Could you check a few things on this model? Use its own coordinates, in mm. A direction names the side the tool comes from. Coordinates: 2 decimals unless noted, no trailing zeros. Order: outer loops, then holes, each group sorted by start corner. A loop starts at its lowest first (then second) coordinate and runs counter-clockwise, first axis right, second up. Notation, with made-up numbers: (-2.75, -17) - (35.25, -17) arc R18 cw to (35.25, 17) - close; hole circle Ø7 at (3, -30.5). An arc over 180 degrees is marked (long way). One line per item, written item: value.
from build123d import *

# Parameters (mm, degrees)
SKETCH1_R           = 5.1435
BOSS_EXTRUDE1_DEPTH = 10.3
BOSS_EXTRUDE2_DEPTH = 7.5
SKETCH3_R           = 10.75
BOSS_EXTRUDE3_DEPTH = 10.3
SKETCH4_R           = 9.525
BOSS_EXTRUDE4_DEPTH = 1.5
SKETCH5_R           = 8.255
BOSS_EXTRUDE5_DEPTH = 12
SKETCH6_R           = 10
BOSS_EXTRUDE6_DEPTH = 11.4
SKETCH7_R           = 4.3053
CUT_EXTRUDE1_DEPTH  = 11.4
SKETCH28_R          = 4.3053
BOSS_EXTRUDE7_DEPTH = 11.4
SKETCH29_R          = 1.5
CUT_EXTRUDE2_DEPTH  = 11.4
CUT_EXTRUDE6_START  = -10.638
SKETCH30_R          = 9.525
CUT_EXTRUDE6_DEPTH  = 10.638
SKETCH31_W          = 0.381
SKETCH31_H          = 3.44369911
SKETCH31_W_2        = 3.44369911
SKETCH31_H_2        = 0.381
BOSS_EXTRUDE8_DEPTH = 7.239
CUT_EXTRUDE7_DEPTH  = 6.731
CUT_EXTRUDE8_DEPTH  = 1.651
CUT_EXTRUDE9_DEPTH  = 1.651
SKETCH35_R          = 9.525
BOSS_EXTRUDE9_DEPTH = 6.731


with BuildPart() as part:
    # Sketch1 → Boss-Extrude1 (new body)
    with BuildSketch(Plane(origin=(0, 0, 0), x_dir=(1, 0, 0), z_dir=(0, 1, 0))):
        with Locations(Location((0, 0, 0), (0, 0, 90))):
            Circle(SKETCH1_R)
    extrude(amount=BOSS_EXTRUDE1_DEPTH)

    # Sketch2 → Boss-Extrude2 (add)
    with BuildSketch(Plane(origin=(0, 10.3, 0), x_dir=(1, 0, 0), z_dir=(0, 1, 0))):
        Polygon((6.206515394, 10.75), (-6.206515394, 10.75), (-12.413030788, 0), (-6.206515394, -10.75), (6.206515394, -10.75), (12.413030788, 0), align=None)
    extrude(amount=BOSS_EXTRUDE2_DEPTH)

    # Sketch3 → Boss-Extrude3 (add)
    with BuildSketch(Plane(origin=(0, 17.8, 0), x_dir=(1, 0, 0), z_dir=(0, 1, 0))):
        with Locations(Location((0, 0, 0), (0, 0, 270))):
            Circle(SKETCH3_R)
    extrude(amount=BOSS_EXTRUDE3_DEPTH)

    # Sketch4 → Boss-Extrude4 (add)
    with BuildSketch(Plane(origin=(0, 28.1, 0), x_dir=(1, 0, 0), z_dir=(0, 1, 0))):
        with Locations(Location((0, 0, 0), (0, 0, 270))):
            Circle(SKETCH4_R)
    extrude(amount=BOSS_EXTRUDE4_DEPTH)

    # Sketch5 → Boss-Extrude5 (add)
    with BuildSketch(Plane(origin=(0, 29.6, 0), x_dir=(1, 0, 0), z_dir=(0, 1, 0))):
        with Locations(Location((0, 0, 0), (0, 0, 270))):
            Circle(SKETCH5_R)
    extrude(amount=BOSS_EXTRUDE5_DEPTH)

    # Sketch6 → Boss-Extrude6 (add)
    with BuildSketch(Plane(origin=(0, 41.6, 0), x_dir=(1, 0, 0), z_dir=(0, 1, 0))):
        with Locations(Location((0, 0, 0), (0, 0, 270))):
            Circle(SKETCH6_R)
    extrude(amount=BOSS_EXTRUDE6_DEPTH)

    # Sketch7 → Cut-Extrude1 (cut)
    with BuildSketch(Plane.XZ):
        with Locations(Location((0, 0, 0), (0, 0, 270))):
            Circle(SKETCH7_R)
    extrude(amount=-CUT_EXTRUDE1_DEPTH, mode=Mode.SUBTRACT)

    # Sketch28 → Boss-Extrude7 (add)
    with BuildSketch(Plane(origin=(0, 0, 0), x_dir=(-1, 0, 0), z_dir=(0, -1, 0))):
        Circle(SKETCH28_R)
    extrude(amount=-BOSS_EXTRUDE7_DEPTH)

    # Sketch29 → Cut-Extrude2 (cut)
    with BuildSketch(Plane.XZ):
        with Locations(Location((0, 0, 0), (0, 0, 270))):
            Circle(SKETCH29_R)
    extrude(amount=-CUT_EXTRUDE2_DEPTH, mode=Mode.SUBTRACT)

    # Sketch30 → Cut-Extrude6 (cut)
    with BuildSketch(Plane(origin=(0, 53, 0), x_dir=(1, 0, 0), z_dir=(0, 1, 0)).offset(CUT_EXTRUDE6_START)):
        with Locations(Location((0, 0, 0), (0, 0, 270))):
            Circle(SKETCH30_R)
    extrude(amount=CUT_EXTRUDE6_DEPTH, mode=Mode.SUBTRACT)

    # Sketch31 → Boss-Extrude8 (add)
    with BuildSketch(Plane(origin=(0, 42.362, 0), x_dir=(1, 0, 0), z_dir=(0, 1, 0))):
        with Locations((0, 3.0226)):
            Rectangle(SKETCH31_W, SKETCH31_H)
        with Locations((-2.2352, 0)):
            Rectangle(SKETCH31_W_2, SKETCH31_H_2)
        with Locations((2.2352, 0)):
            Rectangle(SKETCH31_W_2, SKETCH31_H_2)
    extrude(amount=BOSS_EXTRUDE8_DEPTH)

    # Sketch32 → Cut-Extrude7 (cut)
    with BuildSketch(Plane.XY.offset(0.1905)):
        Polygon((-3.957049555, 48.5088), (-2.2352, 49.601), (-3.957049555, 49.601), align=None)
        Polygon((-0.513350445, 49.601), (-2.2352, 49.601), (-0.513350445, 48.5088), align=None)
    extrude(amount=-CUT_EXTRUDE7_DEPTH, mode=Mode.SUBTRACT)

    # Sketch33 → Cut-Extrude8 (cut)
    with BuildSketch(Plane.XY.offset(0.1905)):
        Polygon((0.513350445, 48.5088), (2.2352, 49.601), (0.513350445, 49.601), align=None)
        Polygon((3.957049555, 49.601), (2.2352, 49.601), (3.957049555, 48.5088), align=None)
    extrude(amount=-CUT_EXTRUDE8_DEPTH, mode=Mode.SUBTRACT)

    # Sketch34 → Cut-Extrude9 (cut)
    with BuildSketch(Plane(origin=(0.1905, 0, 0), x_dir=(0, 0, -1), z_dir=(1, 0, 0))):
        Polygon((1.300750445, 48.5088), (3.0226, 49.601), (1.300750445, 49.601), align=None)
        Polygon((4.744449555, 49.601), (3.0226, 49.601), (4.744449555, 48.5088), align=None)
    extrude(amount=-CUT_EXTRUDE9_DEPTH, mode=Mode.SUBTRACT)

    # Sketch35 → Boss-Extrude9 (add)
    with BuildSketch(Plane(origin=(0, 42.362, 0), x_dir=(1, 0, 0), z_dir=(0, 1, 0))):
        with Locations(Location((0, 0, 0), (0, 0, 270))):
            Circle(SKETCH35_R)
        with BuildLine():
            ThreePointArc((-4.699, -3.683), (-0.167968835, -5.324730553), (4.363062329, -3.683))
            Line((4.363062329, -3.683), (4.363062329, -2.413))
            Line((4.363062329, -2.413), (5.715, -2.413))
            Line((5.715, -2.413), (5.715, 5.24229274))
            Line((5.715, 5.24229274), (3.860385896, 6.985))
            Line((3.860385896, 6.985), (-3.918948776, 6.985))
            Line((-3.918948776, 6.985), (-5.715, 5.188948776))
            Line((-5.715, 5.188948776), (-5.715, -2.413))
            Line((-5.715, -2.413), (-4.699, -2.413))
            Line((-4.699, -2.413), (-4.699, -3.683))
        make_face(mode=Mode.SUBTRACT)
    extrude(amount=BOSS_EXTRUDE9_DEPTH)


solid = part.part
Item 1: I want a section at C-C on z = -7.75. Please give me the cut outline in (x, y), then the cut area to 3 significant figures.
Conclusion:
outline: (-7.94, 10.3) - (7.94, 10.3) - (7.94, 17.8) - (7.45, 17.8) - (7.45, 28.1) - (5.54, 28.1) - (5.54, 29.6) - (2.84, 29.6) - (2.84, 41.6) - (6.32, 41.6) - (6.32, 53) - (5.54, 53) - (5.54, 49.09) - (-5.54, 49.09) - (-5.54, 53) - (-6.32, 53) - (-6.32, 41.6) - (-2.84, 41.6) - (-2.84, 29.6) - (-5.54, 29.6) - (-5.54, 28.1) - (-7.45, 28.1) - (-7.45, 17.8) - (-7.94, 17.8) - close
area: 458 mm²
Item 2: If I drill on probe 1 along Y at (x, z) = (5.25, -6.5); probe 2 along X at (y, z) = (6.5, 0); probe 3 along X at (y, z) = (51.9, 0) (3 decimals), over which ranges is the centre line in solid material (lowest first)?
Conclusion:
probe 1: 10.3 to 29.6, 41.6 to 49.09
probe 2: -5.14 to -1.5, 1.5 to 5.14
probe 3: -10 to -9.525, 9.525 to 10
Item 3: I want a section at B-B on z = 7. Please give me the cut outline in (x, y).
Conclusion:
outline: (-8.37, 10.3) - (8.37, 10.3) - (8.37, 17.8) - (8.16, 17.8) - (8.16, 28.1) - (6.46, 28.1) - (6.46, 29.6) - (4.38, 29.6) - (4.38, 41.6) - (7.14, 41.6) - (7.14, 53) - (6.46, 53) - (6.46, 49.09) - (-6.46, 49.09) - (-6.46, 53) - (-7.14, 53) - (-7.14, 41.6) - (-4.38, 41.6) - (-4.38, 29.6) - (-6.46, 29.6) - (-6.46, 28.1) - (-8.16, 28.1) - (-8.16, 17.8) - (-8.37, 17.8) - close
Item 4: I want a section at D-D on y = 19. Please give me the cut outline in (x, z).
Conclusion:
outline: circle Ø21.5 at (0, 0)
Item 5: Thinking about a two-plate mould opening in Z: for faces 1 (the face through (0.003, 49.063, -3.871)), 2 (the face through (7.27, 22.88, -7.92)), 3 (the face through (-4, 53, 9)), 4 (the face through (0, 42.362, -1)), which applies, pulls with the +Z half, pulls with the -Z half, needs draft (parallel to the pull), parting line crosses it, or undercut?
Conclusion:
face 1: undercut
face 2: parting line crosses it
face 3: needs draft
face 4: undercut
Item 6: I'm going to push flat-ended pins straight in: pin 1 Ø0.9 at (x, z) = (-10.5, -1) entering from +Y; pin 2 Ø1.5 at (x, y) = (-7, 35.5) entering from -Z; pin 3 Ø1 at (x, z) = (8.5, 4) entering from -Y. Where does each tip first touch, or does it pass through?
Conclusion:
pin 1: y = 28.1
pin 2: z = -5.39
pin 3: y = 10.3
Item 7: I want a section at A-A on y = 13. Please give me the cut outline in (x, z), then the cut area to 3 significant figures.
Conclusion:
outline: (-12.41, 0) - (-6.21, -10.75) - (6.21, -10.75) - (12.41, 0) - (6.21, 10.75) - (-6.21, 10.75) - close
area: 400 mm²
Item 8: For faces 5 (the face through (11, 17.8, 0)), 6 (the face through (5.715, 46, -1)), 7 (the face through (6, 17.8, -10)), 8 (the face through (9.266, 13.998, 5.45)), which set-ups out of +Z, -Z, +X, -X, +Y, -Y let a thin tool reach every point of the face, with its end or its side?
Conclusion:
face 5: +X, +Y
face 6: +Y
face 7: -Z, +X, +Y
face 8: +Z, +X, +Y, -Y
